Solid Edge part; units mm, degrees
sketch "Sketch1" plane through (0, 0, 0) normal (0, -1, 0) x (1, 0, 0)
  line L0 (-65, 50) -> (65, 50)
  line L1 (65, 50) -> (65, -50)
  line L2 (65, -50) -> (-65, -50)
  line L3 (-65, -50) -> (-65, 50)
extrude "Protrusion1" add sketch "Sketch1" along normal blind 2
sketch "Sketch2" plane through (0, -2, 0) normal (0, -1, 0) x (1, 0, 0)
  spline S0 degree 2 poles (-63, 37) (-60.7502, 37.0003) (-58.5004, 37) knots 0 0 0 1 1 1
  arc A0 (-52, 43.5018) -> (-58.5004, 37) centre (-58.5, 43.5) cw
  spline S1 degree 2 poles (-52, 48) (-52.0004, 45.7502) (-52, 43.5018) knots 0 0 0 1 1 1
  line L0 (52, 48) -> (-52, 48)
  spline S2 degree 2 poles (52, 48) (52.0003, 45.7502) (52, 43.5004) knots 0 0 0 1 1 1
  arc A1 (58.5018, 37) -> (52, 43.5004) centre (58.5, 43.5) cw
  spline S3 degree 2 poles (63, 37) (60.7502, 37.0004) (58.5018, 37) knots 0 0 0 1 1 1
  line L1 (63, -37) -> (63, 37)
  spline S4 degree 2 poles (63, -37) (60.7502, -37.0003) (58.5004, -37) knots 0 0 0 1 1 1
  arc A2 (52, -43.5018) -> (58.5004, -37) centre (58.5, -43.5) cw
  spline S5 degree 2 poles (52, -48) (52.0004, -45.7502) (52, -43.5018) knots 0 0 0 1 1 1
  line L2 (-52, -48) -> (52, -48)
  spline S6 degree 2 poles (-52, -48) (-52.0003, -45.7502) (-52, -43.5004) knots 0 0 0 1 1 1
  arc A3 (-58.5018, -37) -> (-52, -43.5004) centre (-58.5, -43.5) cw
  spline S7 degree 2 poles (-63, -37) (-60.7502, -37.0004) (-58.5018, -37) knots 0 0 0 1 1 1
  line L3 (-63, 37) -> (-63, -37)
  line L4 (-65, 50) -> (65, 50)
  line L5 (65, 50) -> (65, -50)
  line L6 (65, -50) -> (-65, -50)
  line L7 (-65, -50) -> (-65, 50)
extrude "ExtrudedProtrusion_4" add sketch "Sketch2" along normal blind 6
sketch "Sketch3" plane through (0, -8, 0) normal (0, -1, 0) x (1, 0, 0)
  circle A0 centre (-58.5, 43.5) radius 4.5
  circle A1 centre (58.5, 43.5) radius 4.5
  circle A2 centre (-58.5, -43.5) radius 4.5
  circle A3 centre (58.5, -43.5) radius 4.5
extrude "ExtrudedCutout_2" cut sketch "Sketch3" against normal blind 6 and the other way blind 48.2496
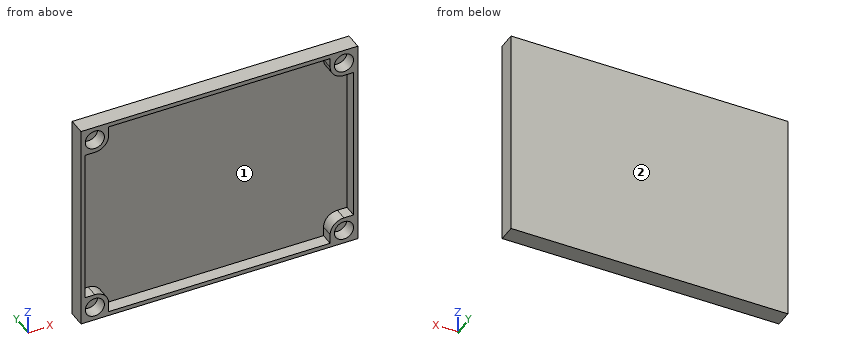
Build history of the part. All positions in model axes, mm. Face numbers are marked on the shaded views. Give positions to 0.01 mm unless a question says otherwise; leave off trailing zeros. Loops run counter-clockwise (first coordinate to the right, second up) from the corner with the lowest first, then second, coordinate; pieces in that order, holes last.
1) Two-plate mould, pull along X, no slides. Class the marked faces 1 and 2: released by +X, released by -X, zero draft, split by the parting line, or undercut.
Values follow:
face 1: undercut
face 2: zero draft
2) Band-saw the part on A-A on x = -6.5. List the corners of the cut face in (y, z).
Values follow:
outline: (-8, -50) - (0, -50) - (0, 50) - (-8, 50) - (-8, 48) - (-2, 48) - (-2, -48) - (-8, -48) - close
3) Band-saw the part on C-C on y = -5. State how many separate pieces and enclosed holes the cut face has, then the cut area to 3 significant figures.
Values follow:
separate pieces: 1
enclosed holes: 5
area: 1,100 mm2
4) Drop a flat-ended pin along its axis: P1, Ø5.5, axis at x = 58.5, z = 43.5, coming from the -Y side. Give the stop position or say it passes through.
Values follow:
P1: stops at y = -2
5) Probe line 1 along Z through (x, y) = (58.5, -5.85); line 2 along Z through (x, y) = (24.5, -4.25); line 3 along X through (y, z) = (-7, 32). List the from-to ranges inside material, lowest first.
Values follow:
line 1: z = -50 to -48, -39 to -37, 37 to 39, 48 to 50
line 2: z = -50 to -48, 48 to 50
line 3: x = -65 to -63, 63 to 65
6) Band-saw the part on B-B on z = -31.5. List the corners of the cut face in (x, y).
Values follow:
outline: (-65, -8) - (-63, -8) - (-63, -2) - (63, -2) - (63, -8) - (65, -8) - (65, 0) - (-65, 0) - close
